Part model, mm, in its own coordinate system. Coordinates: 2 decimals unless noted, no trailing zeros. Order: outer loops, then holes, each group sorted by start corner. A loop starts at its lowest first (then second) coordinate and runs counter-clockwise, first axis right, second up. Notation, with made-up numbers: M 15,-22.5 L 33,-22.5 A11 ccw 33,-8.5 Z; hole C -30,50.25 d1. An arc over 180 degrees is marked long. Answer in a Markdown table with one row per item. Add a question column.
from build123d import *

# Parameters (mm, degrees)
SKETCH1_W           = 171.45
SKETCH1_H           = 304.8
BOSS_EXTRUDE1_DEPTH = 3.175
CUT_EXTRUDE1_DEPTH  = 3.175


with BuildPart() as part:
    # Sketch1 → Boss-Extrude1 (new body)
    with BuildSketch(Plane.XY):
        with Locations((-27.711706949, -64.603096677)):
            Rectangle(SKETCH1_W, SKETCH1_H)
    extrude(amount=BOSS_EXTRUDE1_DEPTH)

    # Sketch2 → Cut-Extrude1 (cut)
    with BuildSketch(Plane.XY.offset(3.175)):
        with BuildLine():
            Line((-59.461706949, -200.003096677), (4.038293051, -200.003096677))
            ThreePointArc((4.038293051, -200.003096677), (7.538293051, -203.503096677), (4.038293051, -207.003096677))
            Line((4.038293051, -207.003096677), (-59.461706949, -207.003096677))
            ThreePointArc((-59.461706949, -207.003096677), (-62.961706949, -203.503096677), (-59.461706949, -200.003096677))
        make_face()
        with BuildLine():
            Line((-59.461706949, -186.003096677), (4.038293051, -186.003096677))
            ThreePointArc((4.038293051, -186.003096677), (7.538293051, -189.503096677), (4.038293051, -193.003096677))
            Line((4.038293051, -193.003096677), (-59.461706949, -193.003096677))
            ThreePointArc((-59.461706949, -193.003096677), (-62.961706949, -189.503096677), (-59.461706949, -186.003096677))
        make_face()
        with BuildLine():
            Line((-59.461706949, -172.003096677), (4.038293051, -172.003096677))
            ThreePointArc((4.038293051, -172.003096677), (7.538293051, -175.503096677), (4.038293051, -179.003096677))
            Line((4.038293051, -179.003096677), (-59.461706949, -179.003096677))
            ThreePointArc((-59.461706949, -179.003096677), (-62.961706949, -175.503096677), (-59.461706949, -172.003096677))
        make_face()
        with BuildLine():
            Line((-59.461706949, -158.003096677), (4.038293051, -158.003096677))
            ThreePointArc((4.038293051, -158.003096677), (7.538293051, -161.503096677), (4.038293051, -165.003096677))
            Line((4.038293051, -165.003096677), (-59.461706949, -165.003096677))
            ThreePointArc((-59.461706949, -165.003096677), (-62.961706949, -161.503096677), (-59.461706949, -158.003096677))
        make_face()
    extrude(amount=-CUT_EXTRUDE1_DEPTH, mode=Mode.SUBTRACT)


solid = part.part
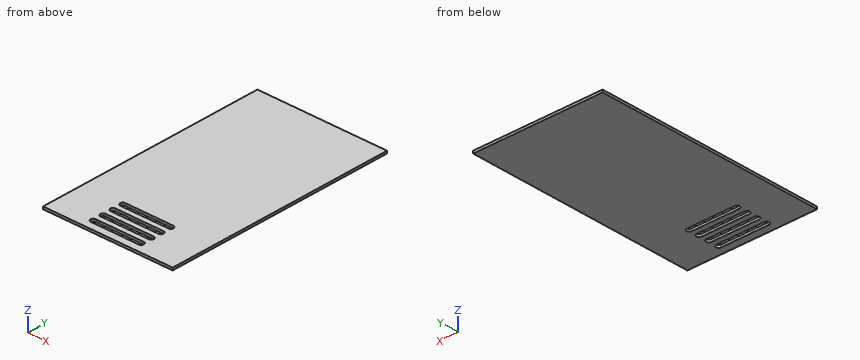
(1) Slice it at B-B (z = 1.65). List the corners of the cut face in (x, y).
(2) Wall check: line 1 (Y direction, x = -22.5, z = 2.8); line 2 (Y direction, x = -62.5, z = 0.55). Give the ranges that are in metal, low to high.
(3) Slice it at A-A (x = -4.5). List the corners of the cut face in (y, z) (3 decimals).
(4) Drop a flat-ended pin along its axis: P1, Ø8, axis at x = -42, y = -44, coming from the -Z side. Give the stop position or say it passes through.
Computed:
| question | item | result |
|---|---|---|
| 1 | outline | M -113.44,-217 L 58.01,-217 L 58.01,87.8 L -113.44,87.8 Z; hole M -59.46,-207 L 4.04,-207 A3.5 ccw 4.04,-200 L -59.46,-200 A3.5 ccw Z; hole M -59.46,-193 L 4.04,-193 A3.5 ccw 4.04,-186 L -59.46,-186 A3.5 ccw Z; hole M -59.46,-179 L 4.04,-179 A3.5 ccw 4.04,-172 L -59.46,-172 A3.5 ccw Z; hole M -59.46,-165 L 4.04,-165 A3.5 ccw 4.04,-158 L -59.46,-158 A3.5 ccw Z |
| 2 | line 1 | y = -217 to -207, -200 to -193, -186 to -179, -172 to -165, -158 to 87.8 |
| 2 | line 2 | y = -217 to -205.24, -201.77 to -191.24, -187.77 to -177.24, -173.77 to -163.24, -159.77 to 87.8 |
| 3 | outline | M -217.003,0 L -207.003,0 L -207.003,3.175 L -217.003,3.175 Z; M -200.003,0 L -193.003,0 L -193.003,3.175 L -200.003,3.175 Z; M -186.003,0 L -179.003,0 L -179.003,3.175 L -186.003,3.175 Z; M -172.003,0 L -165.003,0 L -165.003,3.175 L -172.003,3.175 Z; M -158.003,0 L 87.797,0 L 87.797,3.175 L -158.003,3.175 Z |
| 4 | P1 | stops at z = 0 |
